Geometry: final body of the model. Coordinates: model frame, mm. Give positions to 0.01 mm unless a question says otherwise; leave off trailing zeros. Loops run counter-clockwise (first coordinate to the right, second up) from the corner with the lowest first, then second, coordinate; pieces in that order, holes last. Notation, with made-up numbers: (73, 80) - (103, 80) arc R24 cw to (103, 104) - close; hole circle Ø2 at (77.25, -23.5). An arc over 180 degrees is marked (long way). Answer in a Markdown table with one row per item.
from build123d import *

# Parameters (mm, degrees)
F0_W     = 54
F0_H     = 26
F0_W_2   = 1.5
F0_H_2   = 18
F1_DEPTH = 2


with BuildPart() as f1:
    # F0 (on Right) → F1 (new body)
    with BuildSketch(Plane.YZ):
        with Locations((27, -13)):
            Rectangle(F0_W, F0_H)
        with Locations((5.77, -12)):
            Rectangle(F0_W_2, F0_H_2, mode=Mode.SUBTRACT)
        with Locations((10.49, -12)):
            Rectangle(F0_W_2, F0_H_2, mode=Mode.SUBTRACT)
        with Locations((15.21, -12)):
            Rectangle(F0_W_2, F0_H_2, mode=Mode.SUBTRACT)
        with Locations((19.93, -12)):
            Rectangle(F0_W_2, F0_H_2, mode=Mode.SUBTRACT)
        with Locations((24.65, -12)):
            Rectangle(F0_W_2, F0_H_2, mode=Mode.SUBTRACT)
        with Locations((29.37, -12)):
            Rectangle(F0_W_2, F0_H_2, mode=Mode.SUBTRACT)
        with Locations((34.09, -12)):
            Rectangle(F0_W_2, F0_H_2, mode=Mode.SUBTRACT)
        with Locations((38.81, -12)):
            Rectangle(F0_W_2, F0_H_2, mode=Mode.SUBTRACT)
        with Locations((43.53, -12)):
            Rectangle(F0_W_2, F0_H_2, mode=Mode.SUBTRACT)
        with Locations((48.25, -12)):
            Rectangle(F0_W_2, F0_H_2, mode=Mode.SUBTRACT)
    extrude(amount=F1_DEPTH)


solid = f1.part
Q1. Material intervals for line 1 along Z through (x, y) = (1.55, 29.5), sorted ascending.
Check values:
| item | result |
|---|---|
| line 1 | -26 to -21, -3 to 0 |
Q2. Draft query along Y for faces 1 (the flat face through (1, 0, -13)), 2 (the flat face through (1, 54, -13)), 3 (the flat face through (1, 20, -3)), 4 (the flat face through (1, 19.18, -12)). Return one class per face: pulls with the +Y half, pulls with the -Y half, needs draft (parallel to the pull), parting line crosses it, or undercut.
Check values:
| item | result |
|---|---|
| face 1 | pulls with the -Y half |
| face 2 | pulls with the +Y half |
| face 3 | undercut |
| face 4 | undercut |
Q3. Cut plane A-A (y = 6). Output: boundary loops of the cut face in (x, z).
Check values:
| item | result |
|---|---|
| outline | (0, -26) - (2, -26) - (2, -21) - (0, -21) - close; (0, -3) - (2, -3) - (2, 0) - (0, 0) - close |
Q4. Cut plane B-B (x = 0.75). Give the number of separate pieces and of enclosed holes in the cut face, and give its area (3 significant figures).
Check values:
| item | result |
|---|---|
| separate pieces | 1 |
| enclosed holes | 10 |
| area | 1,130 mm² |
